The listing builds one solid part. Answer for the finished solid, in the listing's coordinates (mm). Face numbers are marked on the shaded views. Round coordinates to 2 decimals unless told otherwise and drop trailing zeros. Loops run counter-clockwise (first coordinate to the right, second up) from the corner with the lowest first, then second, coordinate; pieces in that order, holes last. Notation, with made-up numbers: M 27.5,52 L 84.5,52 A31 ccw 84.5,84 Z; hole C 6.25,-24.75 d4. An arc over 180 degrees is marked long. Answer as a JSON object with one key per item and string values.
```python
from build123d import *

# Parameters (mm, degrees)
F0_W     = 1500
F0_H     = 2000
F1_DEPTH = 100
F3_DEPTH = 100
F4_W     = 60
F4_H     = 1000
F5_DEPTH = 25
F7_R     = 30
F8_DEPTH = 1500.001
F9_R     = 99.99999


# Not quite as in the source:
# - a fillet or chamfer is up to 0.001 mm smaller than in the source, because OpenCascade refuses the exact size


with BuildPart() as f1:
    # F0 (on Front) → F1 (new body)
    with BuildSketch(Plane.XZ):
        with Locations((0.2205967903, 375.376350426)):
            Rectangle(F0_W, F0_H)
    extrude(amount=F1_DEPTH)

    # F2 (on face) → F3 (join)
    with BuildSketch(Plane(origin=(-749.7794032097, 0, 0), x_dir=(0, -1, 0), z_dir=(-1, 0, 0))):
        Polygon((400, 1375.376350426), (100, 1375.376350426), (100, -624.623649574), (300, -624.623649574), (300, 1175.376350426), (400, 1175.376350426), align=None)
    extrude(amount=-F3_DEPTH)

    # F4 (on face) → F5 (cut)
    with BuildSketch(Plane.YZ.offset(-649.7794032097)):
        with Locations((-223.8319441676, -74.623649574)):
            Rectangle(F4_W, F4_H)
    extrude(amount=-F5_DEPTH, mode=Mode.SUBTRACT)

    # F6: F1 across plane


with BuildPart() as f1_1:
    add(f1.part)
    add(f1.part.mirror(Plane.YZ))

    # F7 (on face) → F8 (cut, through all)
    with BuildSketch(Plane(origin=(-749.7794032097, 0, 0), x_dir=(0, -1, 0), z_dir=(-1, 0, 0))):
        with Locations((322.3870694637, 1275.376350426)):
            Circle(F7_R)
    extrude(amount=-F8_DEPTH, mode=Mode.SUBTRACT)

    # F9 (radius 100 in the source; OpenCascade refuses exactly that, so slightly less here)
    f9_edges = [f1_1.edges().sort_by_distance(p)[0] for p in [
        (-699.779403, -400, 1175.37635),
        (699.779403, -400, 1175.37635),
        (-699.779403, -300, -624.62365),
        (699.779403, -300, -624.62365),
        (699.779403, -400, 1375.37635),
        (-699.779403, -400, 1375.37635),
    ]]
    fillet(f9_edges, radius=F9_R)


solid = f1_1.part
```
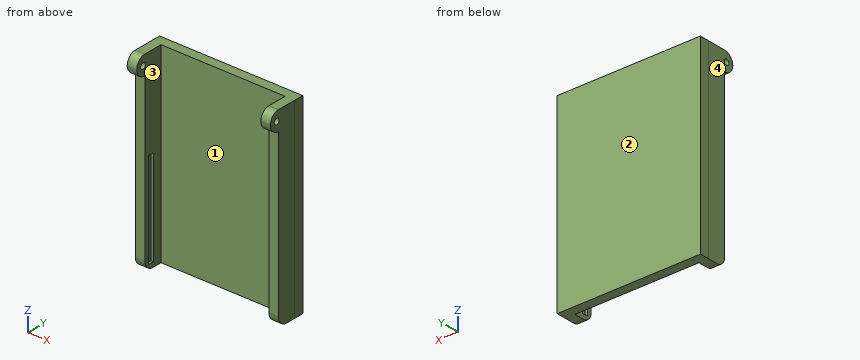
Item 1: The part is cut by section C-C (x = -363.5). Give the vertices of the cut face in (y, z), then the cut area to 3 significant figures.
Values follow:
{"outline": "M -100,-624.62 L 0,-624.62 L 0,1375.38 L -100,1375.38 Z", "area": "200,000 mm^2"}
Item 2: Determine the mould class of the marked faces 1, 2, 3 and 4 for opening direction X: released by +X, released by -X, zero draft, split by the parting line, or undercut.
Values follow:
{"face 1": "undercut", "face 2": "zero draft", "face 3": "undercut", "face 4": "released by -X"}
Item 3: The part is cut by section A-A (y = -172.5). Give the vertices of the cut face in (x, z).
Values follow:
{"outline": "M -749.78,-624.62 L -649.78,-624.62 L -649.78,1375.38 L -749.78,1375.38 Z; M 649.78,-624.62 L 749.78,-624.62 L 749.78,1375.38 L 649.78,1375.38 Z"}
Item 4: The part is cut by section B-B (z = 479.5). Give the vertices of the cut face in (x, y), then the cut area to 3 significant figures.
Values follow:
{"outline": "M -750.22,-100 L -749.78,-100 L -749.78,-300 L -649.78,-300 L -649.78,-100 L 649.78,-100 L 649.78,-300 L 749.78,-300 L 749.78,-100 L 750.22,-100 L 750.22,0 L -750.22,0 Z", "area": "190,000 mm^2"}
Item 5: Straight lines are drawn through the part: line 1 (X direction, y = -139, z = 247.5); line 2 (X direction, y = -207.5, z = 66); line 3 (Y direction, x = 49.5, z = 367.5). For each, find the intervals that lie inside material, in ascending order.
Values follow:
{"line 1": "-749.78 to -649.78, 649.78 to 749.78", "line 2": "-749.78 to -674.78, 674.78 to 749.78", "line 3": "-100 to 0"}
Item 6: The part is cut by section D-D (z = -388.5). Give the vertices of the cut face in (x, y).
Values follow:
{"outline": "M -750.22,-100 L -749.78,-100 L -749.78,-300 L -649.78,-300 L -649.78,-253.83 L -674.78,-253.83 L -674.78,-193.83 L -649.78,-193.83 L -649.78,-100 L 649.78,-100 L 649.78,-193.83 L 674.78,-193.83 L 674.78,-253.83 L 649.78,-253.83 L 649.78,-300 L 749.78,-300 L 749.78,-100 L 750.22,-100 L 750.22,0 L -750.22,0 Z"}
Item 7: Flat-ended cylindrical pins translate along their axes: P1, Ø20, axis at x = 656, z = -34.5, coming from the -Y side; P2, Ø6, axis at x = 464.5, z = 698.5, coming from the +Y side; P3, Ø5, axis at y = -148, z = 934, coming from the -X side; P4, Ø10, axis at y = -155, z = 354, coming from the +X side. Find the tip coordinate at first contact, or state that the pin passes through.
Values follow:
{"P1": "y = -300", "P2": "y = 0", "P3": "x = -749.78", "P4": "x = 749.78"}
